Design review of the part built by this model. Coordinates are the model's own, in mm. Face numbers are marked on the shaded views. Coordinates: 2 decimals unless noted, no trailing zeros. Write each loop counter-clockwise with the first axis right and the second up, starting at its lowest first coordinate (ties: lowest second). Pieces come first, ordered by that corner, then holes. Notation, with made-up numbers: (61, 43) -> (112, 43) arc R26 ccw to (112, 71) -> close; hole circle Ø1 at (87, 64.5). An arc over 180 degrees is marked (long way). One line per question, with ' | ' between items. Start each with the question number.
Q1. Add section D-D on z = 30. State the section outline as (x, y) points, and give its area (3 significant figures).
Q2. For P1, Ø3, axis at x = 7, z = -51, coming from the +Y side; P2, Ø8, axis at x = 5, y = -24, coming from the +Z side; P3, Ø4, axis at y = 17.83, z = 8.26, coming from the +X side; P4, Ø1, axis at x = 12.5, y = 19.5, coming from the +Z side, all flat-tipped, find the tip position at first contact; note any pin that passes through.
Q3. Add section B-B on y = 0. State the section outline as (x, z) points.
Q4. Add section A-A on x = 8. State the section outline as (y, z) points, and give its area (3 significant figures).
Q5. Wall thickness on probe 1 along Z at (x, y) = (4.5, -18); probe 2 along X at (y, z) = (30, -59); probe 3 along Z at (x, y) = (1, -8.5): over which ranges is each line inside the solid? List them lowest first.
Q6. Add section C-C on z = 0. State the section outline as (x, y) points, and give its area (3 significant figures).
Q7. Draft analysis for pull direction Y (two halves, no side actions). For the marked faces 1 and 2, state which applies: pulls with the +Y half, pulls with the -Y half, needs draft (parallel to the pull), parting line crosses it, or undercut.
from build123d import *

# Parameters (mm, degrees)
F0_R     = 5
F0_R_2   = 1.8
F1_DEPTH = 5
F0_R_3   = 2.1
F2_DEPTH = 15


with BuildPart() as f1:
    # F0 (on Right) → F1 (new body)
    with BuildSketch(Plane.YZ):
        with BuildLine():
            Line((-30, -75.14885), (30, -75.14885))
            ThreePointArc((30, -75.14885), (37.071068, -72.219918), (40, -65.14885))
            Line((40, -65.14885), (40, 14.85115))
            ThreePointArc((40, 14.85115), (39.238795, 18.677984), (37.071068, 21.922218))
            ThreePointArc((37.071068, 21.922218), (33.826834, 24.089945), (30, 24.85115))
            Line((30, 24.85115), (21.5, 24.85115))
            Line((21.5, 24.85115), (21.5, 4.58134))
            Line((21.5, 4.58134), (-21.5, 4.58134))
            Line((-21.5, 4.58134), (-21.5, 24.85115))
            Line((-21.5, 24.85115), (-30, 24.85115))
            ThreePointArc((-30, 24.85115), (-34.866502, 23.587119), (-38.502722, 20.114582))
            ThreePointArc((-38.502722, 20.114582), (-39.6184, 17.587277), (-40, 14.85115))
            Line((-40, 14.85115), (-40, -65.14885))
            ThreePointArc((-40, -65.14885), (-37.071068, -72.219918), (-30, -75.14885))
        make_face()
        with Locations((-25.14885, -50.3)):
            Circle(F0_R, mode=Mode.SUBTRACT)
        with Locations((25.15115, -50.3)):
            Circle(F0_R, mode=Mode.SUBTRACT)
        with Locations((-25.14885, 0)):
            Circle(F0_R, mode=Mode.SUBTRACT)
        with Locations((25.15115, 0)):
            Circle(F0_R, mode=Mode.SUBTRACT)
        with BuildLine():
            ThreePointArc((30, 24.85115), (33.826834, 24.089945), (37.071068, 21.922218))
            Line((37.071068, 21.922218), (22.960092, 45.175296))
            ThreePointArc((22.960092, 45.175296), (22.312585, 46.022981), (21.5, 46.714025))
            Line((21.5, 46.714025), (21.5, 24.85115))
            Line((21.5, 24.85115), (30, 24.85115))
        make_face()
        with BuildLine():
            Line((-22.966037, 45.213056), (-38.502722, 20.114582))
            ThreePointArc((-38.502722, 20.114582), (-34.866502, 23.587119), (-30, 24.85115))
            Line((-30, 24.85115), (-21.5, 24.85115))
            Line((-21.5, 24.85115), (-21.5, 46.733685))
            ThreePointArc((-21.5, 46.733685), (-22.314233, 46.05167), (-22.966037, 45.213056))
        make_face()
        with BuildLine():
            Line((13.694858, 24.85115), (21.5, 24.85115))
            Line((21.5, 24.85115), (21.5, 46.714025))
            ThreePointArc((21.5, 46.714025), (20.158098, 47.359594), (18.685587, 47.58134))
            Line((18.685587, 47.58134), (-18.714676, 47.58134))
            ThreePointArc((-18.714676, 47.58134), (-20.170401, 47.364735), (-21.5, 46.733685))
            Line((-21.5, 46.733685), (-21.5, 24.85115))
            Line((-21.5, 24.85115), (-13.694858, 24.85115))
            ThreePointArc((-13.694858, 24.85115), (-0.615713, 39.817548), (13.75, 26.08134))
            ThreePointArc((13.75, 26.08134), (13.736208, 25.465628), (13.694858, 24.85115))
        make_face()
        with Locations((-17.825069, 43.906409)):
            Circle(F0_R_2, mode=Mode.SUBTRACT)
        with Locations((17.825069, 43.906409)):
            Circle(F0_R_2, mode=Mode.SUBTRACT)
        with BuildLine():
            Line((21.5, 4.58134), (21.5, 24.85115))
            Line((21.5, 24.85115), (13.694858, 24.85115))
            ThreePointArc((13.694858, 24.85115), (0, 12.33134), (-13.694858, 24.85115))
            Line((-13.694858, 24.85115), (-21.5, 24.85115))
            Line((-21.5, 24.85115), (-21.5, 4.58134))
            Line((-21.5, 4.58134), (21.5, 4.58134))
        make_face()
        with Locations((-17.825069, 8.256271)):
            Circle(F0_R_2, mode=Mode.SUBTRACT)
        with Locations((17.825069, 8.256271)):
            Circle(F0_R_2, mode=Mode.SUBTRACT)
    extrude(amount=F1_DEPTH)

    # F0 (on Right) → F2 (join)
    with BuildSketch(Plane.YZ):
        with Locations((-25.14885, 0)):
            Circle(F0_R)
        with Locations((-25.14885, 0)):
            Circle(F0_R_3, mode=Mode.SUBTRACT)
        with Locations((25.15115, 0)):
            Circle(F0_R)
        with Locations((25.15115, 0)):
            Circle(F0_R_3, mode=Mode.SUBTRACT)
        with Locations((25.15115, -50.3)):
            Circle(F0_R)
        with Locations((25.15115, -50.3)):
            Circle(F0_R_3, mode=Mode.SUBTRACT)
        with Locations((-25.14885, -50.3)):
            Circle(F0_R)
        with Locations((-25.14885, -50.3)):
            Circle(F0_R_3, mode=Mode.SUBTRACT)
    extrude(amount=F2_DEPTH)


solid = f1.part
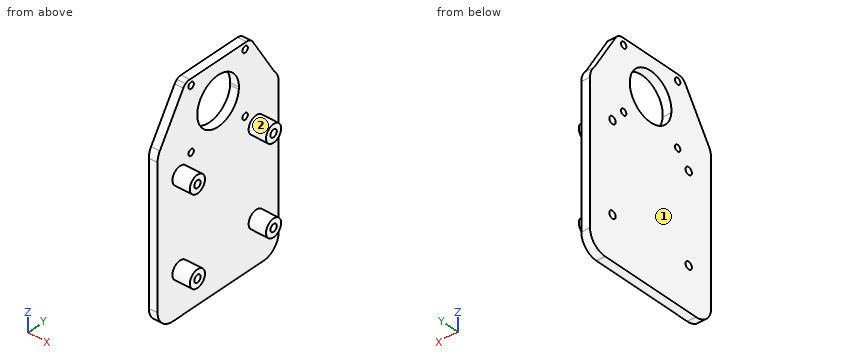
Output values:
1) outline: (0, -32.38) -> (5, -32.38) -> (5, -13.18) -> (0, -13.18) -> close; (0, 13.18) -> (5, 13.18) -> (5, 32.17) -> (0, 32.17) -> close | area: 191 mm2
2) P1: stops at y = 30.15 | P2: stops at z = 47.41 | P3: stops at x = 5 | P4: passes through
3) outline: (0, -75.15) -> (5, -75.15) -> (5, 12.33) -> (0, 12.33) -> close; (0, 39.83) -> (5, 39.83) -> (5, 47.58) -> (0, 47.58) -> close
4) outline: circle Ø10 at (-25.15, -50.3); circle Ø10 at (-25.15, 0); circle Ø10 at (25.15, -50.3); circle Ø10 at (25.15, 0); hole circle Ø4.2 at (-25.15, -50.3); hole circle Ø4.2 at (-25.15, 0); hole circle Ø4.2 at (25.15, -50.3); hole circle Ø4.2 at (25.15, 0) | area: 259 mm2
5) probe 1: z = -75.15 to 6.46, 10.05 to 42.11, 45.7 to 47.58 | probe 2: x = 0 to 5 | probe 3: z = -75.15 to 15.27, 36.89 to 47.58
6) outline: (0, -40) -> (5, -40) -> (5, -30.15) -> (15, -30.15) -> (15, -27.25) -> (0, -27.25) -> close; (0, -23.05) -> (15, -23.05) -> (15, -20.15) -> (5, -20.15) -> (5, 20.15) -> (15, 20.15) -> (15, 23.05) -> (0, 23.05) -> close; (0, 27.25) -> (15, 27.25) -> (15, 30.15) -> (5, 30.15) -> (5, 40) -> (0, 40) -> close | area: 474 mm2
7) face 1: needs draft | face 2: undercut
